Could you check a few things on this model? Use its own coordinates, in mm. A direction names the side the tool comes from. Coordinates: 2 decimals unless noted, no trailing zeros. Write each loop counter-clockwise with the first axis right and the second up, starting at its lowest first coordinate (ties: lowest second). Pieces come first, ordered by that corner, then holes.
Autodesk Inventor part; units mm, degrees
ref_plane "YZ Plane" through (0, 0, 0) normal (1, 0, 0) x (0, 1, 0)
ref_plane "XZ Plane" through (0, 0, 0) normal (0, 1, 0) x (-1, 0, 0)
ref_plane "XY Plane" through (0, 0, 0) normal (0, 0, 1) x (1, 0, 0)
sketch "Sketch1" plane through (0, 0, 0) normal (0, 1, 0) x (-1, 0, 0)
  line L0 (0, 0) -> (140, 0)
  line L1 (140, 0) -> (140, 80)
  line L2 (140, 80) -> (0, 80)
  line L3 (0, 80) -> (0, 0)
  dimension "d0" = 140
  dimension "d1" = 80
extrude "Extrusion2" add sketch "Sketch1" against normal blind 15
sketch "Sketch2" plane through (0, 0, 80) normal (1, 0, 0) x (0, 0, -1)
  line L0 (0, -15) -> (80, -15)
  line L1 (5, -5) -> (28.1523, -5)
  line L2 (28.1523, -5) -> (28.1523, -15)
  line L3 (5, -5) -> (5, -15)
  line L4 (80, 0) -> (80, -15)
  line L5 (0, 0) -> (0, -15)
  line L6 (0, 0) -> (80, 0)
  dimension "d6" = 5
  dimension "d7" = 5
  dimension "d8" = 51.8477
extrude "Extrusion3" cut sketch "Sketch2" against normal through all contours L3 L1 L2 L0
sketch "Sketch3" plane through (0, -15, 0) normal (0, -1, 0) x (1, 0, 0)
  line L0 (0, 51.8477) -> (-140, 51.8477)
  line L1 (-140, 51.8477) -> (-140, 0)
  line L2 (-140, 0) -> (0, 0)
  line L3 (0, 0) -> (0, 51.8477)
  line L4 (-5, 5) -> (-135, 5)
  line L5 (-135, 5) -> (-135, 46.8477)
  line L6 (-135, 46.8477) -> (-5, 46.8477)
  line L7 (-5, 46.8477) -> (-5, 5)
  dimension "d11" = 5
extrude "Electronics_Housing" cut sketch "Sketch3" against normal blind 10 contours L4 L5 L6 L7
sketch "Sketch4" plane through (0, 0, 0) normal (0, 1, 0) x (1, 0, 0)
  circle A0 centre (-110, -63.0196) radius 2
  line L0 (0, 0) -> (-140, 0)
  line L1 (-70, 0) -> (-70, -80) construction
  line L2 (0, -80) -> (-140, -80)
  circle A1 centre (-30, -63.0196) radius 2
  dimension "d14" = 40
  dimension "d15" = 4
extrude "M4_Litho_Holder" cut sketch "Sketch4" against normal through all
sketch "Litho_Dimension" plane through (0, 0, 0) normal (0, 1, 0) x (1, 0, 0)
  line L0 (0, 0) -> (-140, 0)
  line L1 (-140, 0) -> (-140, -80)
  arc A0 (-140, -38.7298) -> (0.3875, -38.0211) centre (-70, 0) ccw construction
  line L2 (-140, -80) -> (0, -80)
sketch "Sketch6" plane through (0, -15, 0) normal (0, -1, 0) x (1, 0, 0)
  line L0 (0, 80) -> (0, 0)
  line L1 (-5, 46.8477) -> (-5, 5)
  line L2 (0, 15.9239) -> (-5, 15.9239)
  line L3 (-5, 15.9239) -> (-5, 35.9239)
  line L4 (-5, 35.9239) -> (0, 35.9239)
  line L5 (0, 35.9239) -> (0, 15.9239)
  line L6 (-140, 0) -> (0, 0)
  line L7 (0, 51.8477) -> (-140, 51.8477)
  point P0 (0, 35.9239)
  dimension "d18" = 15.9238
  dimension "d19" = 20
  dimension "d20" = 15.9238
extrude "ARd_Nano_Mount" cut sketch "Sketch6" against normal blind 5
sketch "Sketch7" plane through (0, 0, 0) normal (0, 1, 0) x (1, 0, 0)
  line L0 (-140, -80) -> (0, -80) construction
  line L1 (-140, -80) -> (-134, -80)
  line L2 (-134, -80) -> (-134, -74)
  line L3 (-134, -74) -> (-140, -74)
  line L4 (-140, -74) -> (-140, -80)
  line L5 (-140, 0) -> (-140, -80)
  line L6 (0, -80) -> (0, 0)
  line L7 (-138, -74) -> (-138, -78)
  line L8 (-138, -78) -> (-134, -78)
  line L9 (-136, -74) -> (-136, -76)
  line L10 (-136, -76) -> (-134, -76)
  line L11 (-70, -80) -> (-70, 0) construction
  line L12 (0, 0) -> (-140, 0)
  line L13 (-140, -40) -> (0, -40) construction
  line L14 (0, -80) -> (-6, -80)
  line L15 (-6, -80) -> (-6, -74)
  line L16 (-6, -74) -> (0, -74)
  line L17 (0, -74) -> (0, -80)
  line L18 (-2, -74) -> (-2, -78)
  line L19 (-2, -78) -> (-6, -78)
  line L20 (-4, -74) -> (-4, -76)
  line L21 (-4, -76) -> (-6, -76)
  line L22 (-140, 0) -> (-134, 0)
  line L23 (-134, 0) -> (-134, -6)
  line L24 (-134, -6) -> (-140, -6)
  line L25 (-140, -6) -> (-140, 0)
  line L26 (-138, -6) -> (-138, -2)
  line L27 (-138, -2) -> (-134, -2)
  line L28 (-136, -6) -> (-136, -4)
  line L29 (-136, -4) -> (-134, -4)
  line L30 (-6, 0) -> (-6, -6)
  line L31 (-4, -6) -> (-4, -4)
  line L32 (-4, -4) -> (-6, -4)
  line L33 (-2, -6) -> (-2, -2)
  line L34 (0, 0) -> (-6, 0)
  line L35 (-6, -6) -> (0, -6)
  line L36 (0, -6) -> (0, 0)
  line L37 (-2, -2) -> (-6, -2)
  point P0 (0, -6)
  dimension "d27" = 2
  dimension "d29" = 2
  dimension "d30" = 2
extrude "Extrusion7" add sketch "Sketch7" along normal blind 99.7 contours L4 L3 L7 L8 L2 L1 | L6 L14 L15 L19 L18 L16 | L12 L6 L35 L33 L37 L30 | L5 L12 L23 L27 L26 L24 | L10 L9 L3 L2 | L28 L29 L23 L24 | L32 L31 L35 L30 | L20 L21 L15 L16
equation "\"d18\" = d20"
properties part number "NL housing_Main"
1. I want a section at C-C on x = -104.5. Please give me the cut outline in (y, z).
Verdict:
outline: (-15, 0) - (0, 0) - (0, 80) - (-15, 80) - (-15, 75) - (-5, 75) - (-5, 51.85) - (-15, 51.85) - (-15, 46.85) - (-5, 46.85) - (-5, 5) - (-15, 5) - close
2. I want a section at A-A on x = -30. Please give me the cut outline in (y, z), plus the area to 3 significant figures.
Verdict:
outline: (-15, 0) - (0, 0) - (0, 61.02) - (-5, 61.02) - (-5, 51.85) - (-15, 51.85) - (-15, 46.85) - (-5, 46.85) - (-5, 5) - (-15, 5) - close; (-15, 75) - (-5, 75) - (-5, 65.02) - (0, 65.02) - (0, 80) - (-15, 80) - close
area: 530 mm2
3. I want a section at B-B on z = 28. Please give me the cut outline in (x, y), plus the area to 3 significant figures.
Verdict:
outline: (-140, -15) - (-135, -15) - (-135, -5) - (-5, -5) - (-5, -10) - (0, -10) - (0, 0) - (-140, 0) - close
area: 775 mm2
4. For pin 1 (5 mm diameter, centred on x = -110, z = 63.02, fed in from -Y); pin 2 (5 mm diameter, centred on x = -60.5, z = 26.5, fed in from +Y), each with a flat end and sliding along its axis, tell me the tip position at first contact or that it passes through.
Verdict:
pin 1: stops at y = -5
pin 2: stops at y = 0
5. Please list where these lines run through material, in increasing order: line 1 along Z through (x, y) = (-110, -2.45); line 2 along X through (y, z) = (16.5, 76.5); line 3 along Y through (x, z) = (-31.5, 47.5).
Verdict:
line 1: z = 0 to 61.02, 65.02 to 80
line 2: x = -140 to -138, -2 to 0
line 3: y = -15 to 0
6. If we mould it in two halves opening along Z, with no side actions, what happens to faces 6 (the face through (-80, -4, 0)), 7 (the face through (-3, -10, 26)), 8 (the face through (-69, -15, 78))? For each: pulls with the +Z half, pulls with the -Z half, needs draft (parallel to the pull), parting line crosses it, or undercut.
Verdict:
face 6: pulls with the -Z half
face 7: undercut
face 8: needs draft
7. On a 3-axis mill with a long thin cutter (end or side, diameter ignored), from which of +Z, -Z, +X, -X, +Y, -Y can I reach the whole of each face in a straight line? I mean faces 1 (the face through (0, -4, 40)), 2 (the face through (-71, -10, 46.848)), 3 (the face through (-3, -13, 35.924)), 4 (the face through (-69, -10, 51.848)), 5 (the face through (-2, 49, 4)). Say none if no direction works.
Verdict:
face 1: +Z, -Z, +X, +Y, -Y
face 2: -Y
face 3: +X, -Y
face 4: +X, -X, -Y
face 5: +Y
8. I want a section at D-D on y = 43. Give the number of separate pieces and of enclosed holes in the cut face, plus the area to 3 significant figures.
Verdict:
separate pieces: 8
enclosed holes: 0
area: 96.0 mm2
